```python
from build123d import *

# Parameters (mm, degrees)
SKETCH1_W           = 25.4
SKETCH1_H           = 25.4
SKETCH1_W_2         = 19.05
SKETCH1_H_2         = 19.05
BOSS_EXTRUDE2_DEPTH = 165.1
CUT_EXTRUDE1_REACH  = 170.963


with BuildPart() as part:
    # Sketch1 → Boss-Extrude2 (new body)
    with BuildSketch(Plane.XY):
        with Locations((12.7, 12.7)):
            Rectangle(SKETCH1_W, SKETCH1_H)
        with Locations((12.7, 12.7)):
            Rectangle(SKETCH1_W_2, SKETCH1_H_2, mode=Mode.SUBTRACT)
    extrude(amount=BOSS_EXTRUDE2_DEPTH)

    # Cut-Extrude1: up to this face of the body (flat: up to its plane)
    cut_extrude1_end = Plane(part.part.faces().sort_by_distance((0, 12.7, 82.55))[0])
    # Sketch3 → Cut-Extrude1 (cut, up to the picked face)
    with BuildSketch(Plane(origin=(25.4, 0, 0), x_dir=(0, 0, -1), z_dir=(1, 0, 0)), mode=Mode.PRIVATE) as cut_extrude1_sk1:
        Polygon((-165.1, 0), (-154.516596402, 25.4), (-165.1, 25.4), align=None)
    cut_extrude1_tool1 = split(extrude(cut_extrude1_sk1.sketch, amount=-CUT_EXTRUDE1_REACH, mode=Mode.PRIVATE), bisect_by=cut_extrude1_end, keep=Keep.BOTH, mode=Mode.PRIVATE)
    # Sketch3 → Cut-Extrude1 (cut, up to the picked face)
    with BuildSketch(Plane(origin=(25.4, 0, 0), x_dir=(0, 0, -1), z_dir=(1, 0, 0)), mode=Mode.PRIVATE) as cut_extrude1_sk2:
        Polygon((0, 0), (-60.959595279, 25.4), (0, 25.4), align=None)
    cut_extrude1_tool2 = split(extrude(cut_extrude1_sk2.sketch, amount=-CUT_EXTRUDE1_REACH, mode=Mode.PRIVATE), bisect_by=cut_extrude1_end, keep=Keep.BOTH, mode=Mode.PRIVATE)
    add(cut_extrude1_tool1.solids().sort_by(Axis((25.4, 16.933333, 161.572199), (-1, 0, 0)))[0], mode=Mode.SUBTRACT)
    add(cut_extrude1_tool2.solids().sort_by(Axis((25.4, 16.933333, 20.319865), (-1, 0, 0)))[0], mode=Mode.SUBTRACT)


solid = part.part
```
Verification items for the finished model (mm, model axes). A direction names the side the tool comes from. Coordinates: 2 decimals unless noted, no trailing zeros. Write each loop counter-clockwise with the first axis right and the second up, starting at its lowest first coordinate (ties: lowest second). Pieces come first, ordered by that corner, then holes. Notation, with made-up numbers: M 13.5,2.5 L 50.5,2.5 A25 cw 50.5,14.5 Z; hole C -7.5,20 d3. An arc over 180 degrees is marked long. Answer as a JSON object with one key per item and string values. Group by question number.
(1) Release check for a two-part mould opening along X. For faces 3 (the face through (13, 25.4, 107)), 4 (the face through (3.175, 13, 102)), 5 (the face through (0, 13, 100)) record: +X half, -X half, draft (parallel to the pull), parting line (faces both ways), or undercut.
(2) Material ranges on line 1 (X direction, y = 6, z = 44.5) (3 decimals); line 2 (Y direction, x = 5, z = 26.5) (3 decimals), recorded low to high.
(3) Tool access check on faces 1 (the face through (13, 22.225, 104)), 2 (the face through (1.589, 12.522, 159.882)). Record the directions out of +Z, -Z, +X, -X, +Y, -Y that give a thin tool (end or side, any length) a straight path to the whole face; none if there is none.
(4) Cross-section at A-A, the plane x = 19.75. Record the cut outline in (y, z) (3 decimals).
(5) Cross-section at B-B, the plane z = 87.5. Record the cut outline in (x, y) (3 decimals), and give its area (3 significant figures).
(6) Cross-section at D-D, the plane x = 1.5. Record the cut outline in (y, z).
(7) Gauge pin test, flat ends, axial feed: pin 1 (10 mm diameter, centred on x = 22.5, y = 9, fed in from -Z); pin 2 (10 mm diameter, centred on x = 17, y = 22, fed in from +Z); pin 3 (3 mm diameter, centred on x = 13, z = 19, fed in from +Y) (3 decimals). Record the tip position at first contact, or that the pin passes through.
(8) Cross-section at C-C, the plane y = 20. Record the cut outline in (x, z) (3 decimals), and give its area (3 significant figures).
Reply:
{
 "1": {"face 3": "draft", "face 4": "undercut", "face 5": "-X half"},
 "2": {"line 1": "0 to 3.175, 22.225 to 25.4", "line 2": "0 to 3.175"},
 "3": {"face 1": "+Z, -Z", "face 2": "+Z, +X, -X, +Y"},
 "4": {"outline": "M 0,0 L 3.175,7.62 L 3.175,163.777 L 0,165.1 Z; M 22.225,53.34 L 25.4,60.96 L 25.4,154.517 L 22.225,155.84 Z"},
 "5": {"outline": "M 0,0 L 25.4,0 L 25.4,25.4 L 0,25.4 Z; hole M 3.175,3.175 L 22.225,3.175 L 22.225,22.225 L 3.175,22.225 Z", "area": "282 mm²"},
 "6": {"outline": "M 0,0 L 25.4,60.96 L 25.4,154.52 L 0,165.1 Z"},
 "7": {"pin 1": "z = 9.6", "pin 2": "z = 155.84", "pin 3": "y = 3.175"},
 "8": {"outline": "M 0,48 L 3.175,48 L 3.175,156.767 L 0,156.767 Z; M 22.225,48 L 25.4,48 L 25.4,156.767 L 22.225,156.767 Z", "area": "691 mm²"}
}
